The model under review builds one solid part; all positions refer to its coordinate system, in mm. A direction names the side the tool comes from. Coordinates: 2 decimals unless noted, no trailing zeros. Write each loop counter-clockwise with the first axis right and the second up, starting at its lowest first coordinate (ties: lowest second). Pieces come first, ordered by that corner, then holes.
Autodesk Inventor part; units mm, degrees
ref_plane "YZ Plane" through (0, 0, 0) normal (1, 0, 0) x (0, 1, 0)
ref_plane "XZ Plane" through (0, 0, 0) normal (0, 1, 0) x (-1, 0, 0)
ref_plane "XY Plane" through (0, 0, 0) normal (0, 0, 1) x (1, 0, 0)
sketch "Sketch2" plane through (0, 0, 0) normal (0, 1, 0) x (-1, 0, 0)
  line L0 (0, 0) -> (0, 40)
  line L1 (0, 40) -> (17.825, 40)
  line L2 (0, 40) -> (0, 46) construction
  line L3 (0, 46) -> (37.5, 46)
  line L4 (21, 36.825) -> (21, 0)
  line L5 (38.5, 45) -> (38.5, 41)
  line L6 (37.5, 40) -> (27, 40)
  line L7 (27, 40) -> (27, 16)
  line L8 (27, 16) -> (37.5, 16)
  line L9 (38.5, 15) -> (38.5, 11)
  line L10 (37.5, 10) -> (27, 10)
  line L11 (27, 10) -> (27, 0)
  line L12 (0, 0) -> (21, 0)
  line L13 (27, 28) -> (38.5, 28)
  arc A0 (21, 36.825) -> (17.825, 40) centre (17.825, 36.825) ccw
  arc A1 (38.5, 45) -> (37.5, 46) centre (37.5, 45) ccw
  arc A2 (37.5, 40) -> (38.5, 41) centre (37.5, 41) ccw
  arc A3 (38.5, 15) -> (37.5, 16) centre (37.5, 15) ccw
  arc A4 (37.5, 10) -> (38.5, 11) centre (37.5, 11) ccw
  line L14 (0, -40) -> (17.825, -40)
  line L15 (0, -46) -> (37.5, -46)
  line L16 (21, -36.825) -> (21, 0)
  line L17 (38.5, -45) -> (38.5, -41)
  line L18 (37.5, -40) -> (27, -40)
  line L19 (27, -40) -> (27, -16)
  line L20 (27, -16) -> (37.5, -16)
  line L21 (38.5, -15) -> (38.5, -11)
  line L22 (37.5, -10) -> (27, -10)
  line L23 (27, -10) -> (27, 0)
  arc A5 (17.825, -40) -> (21, -36.825) centre (17.825, -36.825) ccw
  arc A6 (37.5, -46) -> (38.5, -45) centre (37.5, -45) ccw
  arc A7 (38.5, -41) -> (37.5, -40) centre (37.5, -41) ccw
  arc A8 (37.5, -16) -> (38.5, -15) centre (37.5, -15) ccw
  arc A9 (38.5, -11) -> (37.5, -10) centre (37.5, -11) ccw
  line L24 (0, 40) -> (-17.825, 40)
  line L25 (0, 46) -> (-37.5, 46)
  line L26 (-21, 36.825) -> (-21, 0)
  line L27 (-38.5, 45) -> (-38.5, 41)
  line L28 (-37.5, 40) -> (-27, 40)
  line L29 (-27, 40) -> (-27, 16)
  line L30 (-27, 16) -> (-37.5, 16)
  line L31 (-38.5, 15) -> (-38.5, 11)
  line L32 (-37.5, 10) -> (-27, 10)
  line L33 (-27, 10) -> (-27, 0)
  arc A10 (-17.825, 40) -> (-21, 36.825) centre (-17.825, 36.825) ccw
  arc A11 (-37.5, 46) -> (-38.5, 45) centre (-37.5, 45) ccw
  arc A12 (-38.5, 41) -> (-37.5, 40) centre (-37.5, 41) ccw
  arc A13 (-37.5, 16) -> (-38.5, 15) centre (-37.5, 15) ccw
  arc A14 (-38.5, 11) -> (-37.5, 10) centre (-37.5, 11) ccw
  line L34 (0, -46) -> (-37.5, -46)
  arc A15 (-38.5, -45) -> (-37.5, -46) centre (-37.5, -45) ccw
  line L35 (-38.5, -45) -> (-38.5, -41)
  arc A16 (-37.5, -40) -> (-38.5, -41) centre (-37.5, -41) ccw
  line L36 (-37.5, -40) -> (-27, -40)
  line L37 (-27, -40) -> (-27, -16)
  line L38 (-27, -16) -> (-37.5, -16)
  arc A17 (-38.5, -15) -> (-37.5, -16) centre (-37.5, -15) ccw
  line L39 (-38.5, -15) -> (-38.5, -11)
  arc A18 (-37.5, -10) -> (-38.5, -11) centre (-37.5, -11) ccw
  line L40 (-37.5, -10) -> (-27, -10)
  line L41 (-27, -10) -> (-27, 0)
  line L42 (-21, -36.825) -> (-21, 0)
  line L43 (0, -40) -> (-17.825, -40)
  arc A19 (-21, -36.825) -> (-17.825, -40) centre (-17.825, -36.825) ccw
  line L44 (23.5, 38) -> (23.5, -46) construction
  point P0 (21, 40)
  point P1 (38.5, 46)
  point P2 (38.5, 40)
  point P3 (38.5, 16)
  point P4 (38.5, 10)
  point P5 (32.74, 41.8)
  point P6 (32.74, 14.2)
  point P7 (32.74, -41.8)
  point P8 (32.74, -14.2)
  point P9 (-32.74, 41.8)
  point P10 (-32.74, 14.2)
  point P11 (-32.74, -41.8)
  point P12 (-32.74, -14.2)
  point P13 (-23.5, 38)
  point P14 (23.5, -38)
  point P15 (23.5, 10)
  point P16 (23.5, 16)
  point P17 (-23.5, 38)
  point P18 (-23.5, -38)
  point P19 (-23.5, 10)
  point P20 (-23.5, 16)
  point P21 (23.5, 0)
  point P22 (-23.5, 0)
  dimension "d2" = 40
  dimension "d3" = 6
  dimension "d4" = 38.5
  dimension "d5" = 21
  dimension "d6" = 6
  dimension "d7" = 11.5
  dimension "d8" = 24
  dimension "d9" = 11.5
  dimension "d10" = 6
  dimension "d11" = 11.5
  dimension "d12" = 5.74
  dimension "d13" = 27.6
  dimension "d14" = 3.175
  dimension "d15" = 1
  dimension "d26" = 8
  dimension "d37" = 47
  dimension "d40" = 22
  dimension "d42" = 48
  dimension "d43" = 6
  dimension "d44" = 46
extrude "Extrusion2" add sketch "Sketch2" along normal blind 10
hole "Hole1" at (-32.74, 0, 41.8) at (-32.74, 0, 14.2) at (-32.74, 0, -41.8) at (-32.74, 0, -14.2) at (32.74, 0, 41.8) at (32.74, 0, 14.2) at (32.74, 0, -14.2) at (32.74, 0, -41.8) direction (0, 1, 0) diameter 1.567 end through all countersink diameter 2.5 countersink angle 90
hole "Hole2" at (-23.5, 0, 38) at (23.5, 0, 38) at (-23.5, 0, 16) at (-23.5, 0, 10) at (-23.5, 0, -38) at (23.5, 0, -38) at (23.5, 0, 16) at (23.5, 0, 10) at (23.5, 0, 0) at (-23.5, 0, 0) direction (0, 1, 0) diameter 2 end through all
properties part number "rapoukBasev5" material "EN AW-6060 T6"
Item 1: Mouldability with a two-part tool opening along Y and no side actions: class faces 1 (the face through (26, 10, 1)), 2 (the face through (-38.5, 5, 13)) as pulls with the +Y half, pulls with the -Y half, needs draft (parallel to the pull), parting line crosses it, or undercut.
Solved:
face 1: pulls with the +Y half
face 2: needs draft
Item 2: Take a section at A-A, the plane x = 28.5. Write out the cut boundary in (y, z).
Solved:
outline: (0, -46) - (10, -46) - (10, -40) - (0, -40) - close; (0, -16) - (10, -16) - (10, -10) - (0, -10) - close; (0, 10) - (10, 10) - (10, 16) - (0, 16) - close; (0, 40) - (10, 40) - (10, 46) - (0, 46) - close
Item 3: Take a section at B-B, the plane x = 13. Write out the cut boundary in (y, z).
Solved:
outline: (0, -46) - (10, -46) - (10, -40) - (0, -40) - close; (0, 40) - (10, 40) - (10, 46) - (0, 46) - close
Item 4: For pin 1 (1.8 mm diameter, centred on x = 32.74, z = -41.8, fed in from +Y); pin 2 (4 mm diameter, centred on y = 5.5, z = 26, fed in from +X); pin 3 (1.2 mm diameter, centred on x = 23.5, z = 38, fed in from +Y); pin 4 (1.8 mm diameter, centred on x = 32.74, z = 14.2, fed in from -Y), all flat-tipped, find the tip position at first contact; note any pin that passes through.
Solved:
pin 1: stops at y = 10
pin 2: stops at x = 27
pin 3: passes through
pin 4: stops at y = 0.35
Item 5: Machinability: for faces 3 (the face through (-38.5, 5, 43)), 4 (the face through (32, 5, 10)), 5 (the face through (-27, 5, 0)), 6 (the face through (20.09, 4.93, 39.05)), which of the approach directions +Z, -Z, +X, -X, +Y, -Y give a long, thin tool a straight path to every point of the face, cutting with its end or side? Answer none if there is none.
Solved:
face 3: +Z, -Z, -X, +Y, -Y
face 4: +X, +Y, -Y
face 5: -X, +Y, -Y
face 6: +Y, -Y
Item 6: Take a section at D-D, the plane z = -38. Write out the cut boundary in (x, y), plus the area to 3 significant figures.
Solved:
outline: (-27, 0) - (-24.5, 0) - (-24.5, 10) - (-27, 10) - close; (-22.5, 0) - (-20.77, 0) - (-20.77, 10) - (-22.5, 10) - close; (20.77, 0) - (22.5, 0) - (22.5, 10) - (20.77, 10) - close; (24.5, 0) - (27, 0) - (27, 10) - (24.5, 10) - close
area: 84.5 mm2
Item 7: Take a section at C-C, the plane z = -21. Write out the cut boundary in (x, y), plus the area to 3 significant figures.
Solved:
outline: (-27, 0) - (-21, 0) - (-21, 10) - (-27, 10) - close; (21, 0) - (27, 0) - (27, 10) - (21, 10) - close
area: 120 mm2
Item 8: To check wall thickness, follow line 1 along Z through (x, y) = (-23.5, 4); line 2 along Z through (x, y) = (18, 6.5); line 3 along X through (y, z) = (4.75, 14). State the ranges of each line that lie inside material, in increasing order.
Solved:
line 1: z = -46 to -39, -37 to -1, 1 to 9, 11 to 15, 17 to 37, 39 to 46
line 2: z = -46 to -40, 40 to 46
line 3: x = -38.5 to -33.5, -31.98 to -21, 21 to 31.98, 33.5 to 38.5
